Check sheet for the modelled part. Datum: model origin and axes. Units: mm. Face numbers are marked on the shaded views. A direction names the side the tool comes from. Round coordinates to 2 decimals unless told otherwise and drop trailing zeros. Write each loop counter-clockwise with the first axis right and the second up, starting at its lowest first coordinate (ties: lowest second). Pieces come first, ordered by that corner, then holes. Notation, with made-up numbers: M 28,18 L 55,18 A22 ccw 55,33 Z; hole C 32.25,-28 d7. An arc over 180 degrees is marked long. Answer in a Markdown table with one row per item.
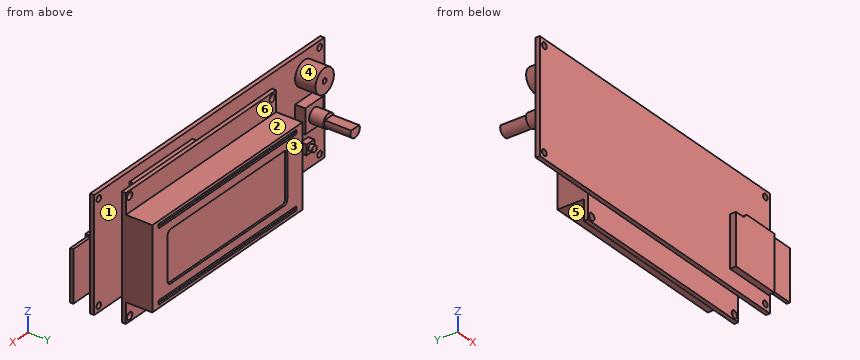
```python
from build123d import *

# Parameters (mm, degrees)
SKETCH1_W           = 150
SKETCH1_H           = 55
SKETCH1_R           = 1.5
BOSS_EXTRUDE1_DEPTH = 2
SKETCH2_R           = 6
BOSS_EXTRUDE2_DEPTH = 10
SKETCH3_W           = 12
SKETCH3_H           = 12
BOSS_EXTRUDE3_DEPTH = 25
SKETCH4_W           = 5
SKETCH4_H           = 5
SKETCH4_W_2         = 41
SKETCH4_H_2         = 3
BOSS_EXTRUDE4_DEPTH = 5
SKETCH5_W           = 41
SKETCH5_H           = 3
SKETCH5_W_2         = 5
SKETCH5_H_2         = 5
SKETCH5_R           = 1.5
CUT_EXTRUDE1_DEPTH  = 2
SKETCH6_W           = 12
SKETCH6_H           = 12
CUT_EXTRUDE2_DEPTH  = 13
SKETCH7_W           = 12
SKETCH7_H           = 12
SKETCH7_R           = 3.5
CUT_EXTRUDE3_DEPTH  = 7
SKETCH8_R           = 1.25
CUT_EXTRUDE4_DEPTH  = 5
BOSS_EXTRUDE5_DEPTH = 3
SKETCH10_W          = 25
SKETCH10_H          = 1.5
CUT_EXTRUDE5_DEPTH  = 18
SKETCH11_W          = 98
SKETCH11_H          = 60
SKETCH11_R          = 1.75
BOSS_EXTRUDE6_DEPTH = 2
SKETCH12_W          = 98
SKETCH12_H          = 40
BOSS_EXTRUDE7_DEPTH = 13
CUT_EXTRUDE6_DEPTH  = 1
SKETCH14_W          = 25
SKETCH14_H          = 1.5
BOSS_EXTRUDE8_DEPTH = 29


with BuildPart() as part:
    # Sketch1 → Boss-Extrude1 (new body)
    with BuildSketch(Plane(origin=(0, 0, 0), x_dir=(1, 0, 0), z_dir=(0, 1, 0))):
        with Locations((75, 27.5)):
            Rectangle(SKETCH1_W, SKETCH1_H)
        with Locations((3, 52)):
            Circle(SKETCH1_R, mode=Mode.SUBTRACT)
        with Locations((147, 52)):
            Circle(SKETCH1_R, mode=Mode.SUBTRACT)
        with Locations((147, 3)):
            Circle(SKETCH1_R, mode=Mode.SUBTRACT)
        with Locations((3, 3)):
            Circle(SKETCH1_R, mode=Mode.SUBTRACT)
    extrude(amount=BOSS_EXTRUDE1_DEPTH)

    # Sketch2 → Boss-Extrude2 (add)
    with BuildSketch(Plane(origin=(0, 2, 0), x_dir=(1, 0, 0), z_dir=(0, 1, 0))):
        with Locations((13, 10)):
            Circle(SKETCH2_R)
    extrude(amount=BOSS_EXTRUDE2_DEPTH)

    # Sketch3 → Boss-Extrude3 (add)
    with BuildSketch(Plane(origin=(0, 2, 0), x_dir=(1, 0, 0), z_dir=(0, 1, 0))):
        with Locations((13, 27.5)):
            Rectangle(SKETCH3_W, SKETCH3_H)
    extrude(amount=BOSS_EXTRUDE3_DEPTH)

    # Sketch4 → Boss-Extrude4 (add)
    with BuildSketch(Plane(origin=(0, 2, 0), x_dir=(1, 0, 0), z_dir=(0, 1, 0))):
        with Locations((13, 43)):
            Rectangle(SKETCH4_W, SKETCH4_H)
        with Locations((106.5, 6.5)):
            Rectangle(SKETCH4_W_2, SKETCH4_H_2)
    extrude(amount=BOSS_EXTRUDE4_DEPTH)

    # Sketch5 → Cut-Extrude1 (cut)
    with BuildSketch(Plane(origin=(0, 7, 0), x_dir=(1, 0, 0), z_dir=(0, 1, 0))):
        with Locations((106.5, 6.5)):
            Rectangle(SKETCH5_W, SKETCH5_H)
        with Locations((13, 43)):
            Rectangle(SKETCH5_W_2, SKETCH5_H_2)
        with Locations((13, 43)):
            Circle(SKETCH5_R, mode=Mode.SUBTRACT)
    extrude(amount=-CUT_EXTRUDE1_DEPTH, mode=Mode.SUBTRACT)

    # Sketch6 → Cut-Extrude2 (cut)
    with BuildSketch(Plane(origin=(0, 27, 0), x_dir=(1, 0, 0), z_dir=(0, 1, 0))):
        with Locations((13, 27.5)):
            Rectangle(SKETCH6_W, SKETCH6_H)
        with BuildLine():
            Line((10.370614338, 26.055586264), (15.629385662, 26.055586264))
            ThreePointArc((15.629385662, 26.055586264), (13, 30.5), (10.370614338, 26.055586264))
        make_face(mode=Mode.SUBTRACT)
    extrude(amount=-CUT_EXTRUDE2_DEPTH, mode=Mode.SUBTRACT)

    # Sketch7 → Cut-Extrude3 (cut)
    with BuildSketch(Plane(origin=(0, 14, 0), x_dir=(1, 0, 0), z_dir=(0, 1, 0))):
        with Locations((13, 27.5)):
            Rectangle(SKETCH7_W, SKETCH7_H)
        with Locations((13, 27.5)):
            Circle(SKETCH7_R, mode=Mode.SUBTRACT)
    extrude(amount=-CUT_EXTRUDE3_DEPTH, mode=Mode.SUBTRACT)

    # Sketch8 → Cut-Extrude4 (cut)
    with BuildSketch(Plane(origin=(0, 12, 0), x_dir=(1, 0, 0), z_dir=(0, 1, 0))):
        with Locations((13, 10)):
            Circle(SKETCH8_R)
    extrude(amount=-CUT_EXTRUDE4_DEPTH, mode=Mode.SUBTRACT)

    # Sketch9 → Boss-Extrude5 (add)
    with BuildSketch(Plane.XZ):
        Polygon((149, -20), (131, -20), (129, -22), (124, -22), (124, -47), (149, -47), align=None)
    extrude(amount=BOSS_EXTRUDE5_DEPTH)

    # Sketch10 → Cut-Extrude5 (cut)
    with BuildSketch(Plane(origin=(149, 0, 0), x_dir=(0, 0, -1), z_dir=(1, 0, 0))):
        with Locations((33.5, -1.5)):
            Rectangle(SKETCH10_W, SKETCH10_H)
    extrude(amount=-CUT_EXTRUDE5_DEPTH, mode=Mode.SUBTRACT)

    # Sketch11 → Boss-Extrude6 (add)
    with BuildSketch(Plane(origin=(0, 5, 0), x_dir=(1, 0, 0), z_dir=(0, 1, 0))):
        with Locations((87, 34)):
            Rectangle(SKETCH11_W, SKETCH11_H)
        with Locations((40.5, 61.5)):
            Circle(SKETCH11_R, mode=Mode.SUBTRACT)
        with Locations((133.5, 61.5)):
            Circle(SKETCH11_R, mode=Mode.SUBTRACT)
        with Locations((133.5, 6.5)):
            Circle(SKETCH11_R, mode=Mode.SUBTRACT)
        with Locations((40.5, 6.5)):
            Circle(SKETCH11_R, mode=Mode.SUBTRACT)
    extrude(amount=BOSS_EXTRUDE6_DEPTH)

    # Sketch12 → Boss-Extrude7 (add)
    with BuildSketch(Plane(origin=(0, 7, 0), x_dir=(1, 0, 0), z_dir=(0, 1, 0))):
        with Locations((87, 34)):
            Rectangle(SKETCH12_W, SKETCH12_H)
    extrude(amount=BOSS_EXTRUDE7_DEPTH)

    # Sketch13 → Cut-Extrude6 (cut)
    with BuildSketch(Plane(origin=(0, 20, 0), x_dir=(1, 0, 0), z_dir=(0, 1, 0))):
        with BuildLine():
            Line((50, 46.5), (124, 46.5))
            ThreePointArc((124, 46.5), (125.414213562, 45.914213562), (126, 44.5))
            Line((126, 44.5), (126, 23.5))
            ThreePointArc((126, 23.5), (125.414213562, 22.085786438), (124, 21.5))
            Line((124, 21.5), (50, 21.5))
            ThreePointArc((50, 21.5), (48.585786438, 22.085786438), (48, 23.5))
            Line((48, 23.5), (48, 44.5))
            ThreePointArc((48, 44.5), (48.585786438, 45.914213562), (50, 46.5))
        make_face()
        with BuildLine():
            Line((42.5, 52.5), (131.5, 52.5))
            ThreePointArc((131.5, 52.5), (131.853553391, 52.353553391), (132, 52))
            Line((132, 52), (132, 51))
            ThreePointArc((132, 51), (131.853553391, 50.646446609), (131.5, 50.5))
            Line((131.5, 50.5), (42.5, 50.5))
            ThreePointArc((42.5, 50.5), (42.146446609, 50.646446609), (42, 51))
            Line((42, 51), (42, 52))
            ThreePointArc((42, 52), (42.146446609, 52.353553391), (42.5, 52.5))
        make_face()
        with BuildLine():
            Line((132, 16), (132, 17))
            ThreePointArc((132, 17), (131.853553391, 17.353553391), (131.5, 17.5))
            Line((131.5, 17.5), (42.5, 17.5))
            ThreePointArc((42.5, 17.5), (42.146446609, 17.353553391), (42, 17))
            Line((42, 17), (42, 16))
            ThreePointArc((42, 16), (42.146446609, 15.646446609), (42.5, 15.5))
            Line((42.5, 15.5), (131.5, 15.5))
            ThreePointArc((131.5, 15.5), (131.853553391, 15.646446609), (132, 16))
        make_face()
    extrude(amount=-CUT_EXTRUDE6_DEPTH, mode=Mode.SUBTRACT)

    # Sketch14 → Boss-Extrude8 (add)
    with BuildSketch(Plane(origin=(131, 0, 0), x_dir=(0, 0, -1), z_dir=(1, 0, 0))):
        with Locations((33.5, -1.5)):
            Rectangle(SKETCH14_W, SKETCH14_H)
    extrude(amount=BOSS_EXTRUDE8_DEPTH)


solid = part.part
```
1. Access from +Z, -Z, +X, -X, +Y, -Y to the whole of each face (thin tool, end or side, straight path). Record for the marked faces 4, 5 and 6.
Found:
| item | result |
|---|---|
| face 4 | +Y |
| face 5 | -Z, +X, -X, +Y |
| face 6 | +Z, +X, +Y |
2. Section check B-B, the plane x = 133.5. Record the cut outline in (y, z).
Found:
| item | result |
|---|---|
| outline | M -3,-47 L 0,-47 L 0,-55 L 2,-55 L 2,0 L 0,0 L 0,-20 L -3,-20 Z; M 5,-64 L 7,-64 L 7,-63.25 L 5,-63.25 Z; M 5,-59.75 L 7,-59.75 L 7,-54 L 20,-54 L 20,-14 L 7,-14 L 7,-8.25 L 5,-8.25 Z; M 5,-4.75 L 7,-4.75 L 7,-4 L 5,-4 Z |
3. Section check A-A, the plane x = 3. Record the cut outline in (y, z).
Found:
| item | result |
|---|---|
| outline | M 0,-55 L 2,-55 L 2,-53.5 L 0,-53.5 Z; M 0,-50.5 L 2,-50.5 L 2,-4.5 L 0,-4.5 Z; M 0,-1.5 L 2,-1.5 L 2,0 L 0,0 Z |
4. Draft check along Y on the marked faces 1, 2 and 3. Enter one of: +Y half, -Y half, draft (parallel to the pull), parting line (faces both ways), or undercut.
Found:
| item | result |
|---|---|
| face 1 | undercut |
| face 2 | draft |
| face 3 | +Y half |
5. Scan lines: L1, parallel to X at y = 1.55, z = -3; L2, parallel to Z at x = 40.5, y = 6.1; L3, parallel to Z at x = 3, y = 0.65. Record each from-to range of solid material in increasing order.
Found:
| item | result |
|---|---|
| L1 | x = 0 to 1.5, 4.5 to 145.5, 148.5 to 150 |
| L2 | z = -64 to -63.25, -59.75 to -8.25, -4.75 to -4 |
| L3 | z = -55 to -53.5, -50.5 to -4.5, -1.5 to 0 |
6. Section check C-C, the plane z = -6.5. Record the cut outline in (x, y), and give its area (3 significant figures).
Found:
| item | result |
|---|---|
| outline | M 0,0 L 150,0 L 150,2 L 127,2 L 127,5 L 131.75,5 L 131.75,7 L 42.25,7 L 42.25,5 L 86,5 L 86,2 L 17.87,2 L 17.87,12 L 8.13,12 L 8.13,2 L 0,2 Z; M 38,5 L 38.75,5 L 38.75,7 L 38,7 Z; M 135.25,5 L 136,5 L 136,7 L 135.25,7 Z |
| area | 702 mm2 |
7. Go/stop test with flat-tipped pins: pin 1 (6 mm diameter, centred on x = 22, z = -48.5, fed in from -Y); pin 2 (4.5 mm diameter, centred on x = 133.5, z = -61.5, fed in from -Y); pin 3 (0.5 mm diameter, centred on y = 19.5, z = -35.5, fed in from +X); pin 4 (2.5 mm diameter, centred on x = 147, z = -52, fed in from -Y). Record where each tip stops, or that it passes through.
Found:
| item | result |
|---|---|
| pin 1 | stops at y = 0 |
| pin 2 | stops at y = 5 |
| pin 3 | stops at x = 136 |
| pin 4 | passes through |
